from build123d import *

# Parameters (mm, degrees)
SKETCH1_W           = 100
SKETCH1_H           = 80
BOSS_EXTRUDE1_DEPTH = 5
SKETCH2_R           = 8.0125
CUT_EXTRUDE1_DEPTH  = 129.16005618
BOSS_EXTRUDE2_START = 45
SKETCH3_R           = 20.715
SKETCH3_R_2         = 8.0125
BOSS_EXTRUDE2_DEPTH = 45
SKETCH4_R           = 2.0193
CUT_EXTRUDE2_DEPTH  = 15
SKETCH6_R           = 2.0193
CUT_EXTRUDE3_DEPTH  = 15
SKETCH7_R           = 7.9375
CUT_EXTRUDE4_DEPTH  = 136.738719638


with BuildPart() as part:
    # Sketch1 → Boss-Extrude1 (new body)
    with BuildSketch(Plane(origin=(0, 0, 0), x_dir=(1, 0, 0), z_dir=(0, 1, 0))):
        with Locations((50, -40)):
            Rectangle(SKETCH1_W, SKETCH1_H)
    extrude(amount=BOSS_EXTRUDE1_DEPTH)

    # Sketch2 → Cut-Extrude1 (cut, through all)
    with BuildSketch(Plane(origin=(0, 5, 0), x_dir=(1, 0, 0), z_dir=(0, 1, 0))):
        with Locations(Location((50, -40, 0), (0, 0, 270))):
            Circle(SKETCH2_R)
    extrude(amount=-CUT_EXTRUDE1_DEPTH, mode=Mode.SUBTRACT)

    # Sketch3 → Boss-Extrude2 (add)
    with BuildSketch(Plane(origin=(0, 5, 0), x_dir=(1, 0, 0), z_dir=(0, 1, 0)).offset(BOSS_EXTRUDE2_START)):
        with Locations(Location((50, -40, 0), (0, 0, 90))):
            Circle(SKETCH3_R)
        with Locations(Location((50, -40, 0), (0, 0, 270))):
            Circle(SKETCH3_R_2, mode=Mode.SUBTRACT)
    extrude(amount=-BOSS_EXTRUDE2_DEPTH)

    # Sketch4 → Cut-Extrude2 (cut)
    with BuildSketch(Plane(origin=(63.180969698, 50, 55.980402461), x_dir=(0.7714411036002745, 0, -0.6363007336755088), z_dir=(0.6363007336755088, 0, 0.7714411036002745))):
        with Locations((0, -10)):
            Circle(SKETCH4_R)
        with Locations((0, -35)):
            Circle(SKETCH4_R)
    extrude(amount=-CUT_EXTRUDE2_DEPTH, mode=Mode.SUBTRACT)

    # Sketch6 → Cut-Extrude3 (cut)
    with BuildSketch(Plane(origin=(52.5543225, 0, -17.601285723), x_dir=(0, -1, 0), z_dir=(0.9482321037380778, 0, -0.3175781438330723))):
        with Locations(Location((-40, -53.808191341, 0), (0, 0, 90))):
            Circle(SKETCH6_R)
        with Locations(Location((-15, -53.808191341, 0), (0, 0, 90))):
            Circle(SKETCH6_R)
    extrude(amount=-CUT_EXTRUDE3_DEPTH, mode=Mode.SUBTRACT)

    # Sketch7 → Cut-Extrude4 (cut, through all)
    with BuildSketch(Plane(origin=(0, 5, 0), x_dir=(1, 0, 0), z_dir=(0, 1, 0))):
        with Locations(Location((84.125, -64.125, 0), (0, 0, 270))):
            Circle(SKETCH7_R)
        with Locations(Location((15.875, -64.125, 0), (0, 0, 270))):
            Circle(SKETCH7_R)
        with Locations(Location((15.875, -15.875, 0), (0, 0, 270))):
            Circle(SKETCH7_R)
        with Locations(Location((84.125, -15.875, 0), (0, 0, 270))):
            Circle(SKETCH7_R)
    extrude(amount=-CUT_EXTRUDE4_DEPTH, mode=Mode.SUBTRACT)


solid = part.part
Can you work these out from the model? Positions are in its coordinate system, mm. A direction names the side the tool comes from. Round coordinates to 2 decimals unless told otherwise and drop trailing zeros. Write each loop counter-clockwise with the first axis right and the second up, starting at its lowest first coordinate (ties: lowest second). Pieces come first, ordered by that corner, then holes. Notation, with made-up numbers: (25.5, 79.25) -> (33.5, 79.25) arc R11 cw to (33.5, 88.25) -> close; hole circle Ø4 at (51, 57). An arc over 180 degrees is marked (long way). One line per question, with ' | ' between items. Start each with the question number.
1) I need wall thicknesses on line 1 (X direction, y = 12.5, z = 40) (1 decimal); line 2 (Z direction, x = 84.5, y = 3); line 3 (Z direction, x = 12.5, y = 3). Which ranges of each line are inside material? Lowest first, please. Write a range as [from, to].
2) Suppose I cut it at A-A on x = 50. Write out the boundary of the cut face in (y, z) (1 decimal).
3) If we mould it in two halves opening along Z, with no side actions, what happens to faces 1 (the cylindrical face through (64.221, 15.089, 37.365)), 2 (the flat face through (49, 2, 0)), 3 (the flat face through (49, 0, 31))? For each: released by +Z, released by -Z, zero draft, split by the parting line, or undercut.
4) I'm going to push flat-ended pins straight in: P1, Ø20.5, axis at x = 84.125, z = 15.875, coming from the +Y side; P2, Ø1, axis at y = 26, z = 52, coming from the -X side; P3, Ø6, axis at y = 24, z = 33, coming from the -X side. Where does each tip first touch, or does it pass through?
5) Suppose I cut it at B-B on z = 10. Write out the boundary of the cut face in (x, y), then the cut area to 3 significant figures.
6) Suppose I cut it at D-D on x = 88. Write out the boundary of the cut face in (y, z).
7) Suppose I cut it at C-C on y = 35.5. Write out the boundary of the cut face in (x, z) (1 decimal).
8) On a 3-axis mill with a long thin cutter (end or side, diameter ignored), from which of +Z, -Z, +X, -X, +Y, -Y can I reach the whole of each face in a straight line? I mean faces 4 (the cylindrical face through (68.378, 27.815, 30.441)), 5 (the flat face through (49, 2, 80)). Say none if no direction works.
Return value:
1) line 1: x = [29.3, 42], [58, 70.7] | line 2: z = [0, 7.95], [23.8, 56.2], [72.05, 80] | line 3: z = [0, 8.69], [23.06, 56.94], [71.31, 80]
2) outline: (0, 0) -> (5, 0) -> (5, 19.3) -> (50, 19.3) -> (50, 32) -> (0, 32) -> close; (0, 48) -> (50, 48) -> (50, 60.7) -> (5, 60.7) -> (5, 80) -> (0, 80) -> close
3) face 1: undercut | face 2: released by -Z | face 3: zero draft
4) P1: stops at y = 5 | P2: stops at x = 32.77 | P3: stops at x = 29.67
5) outline: (0, 0) -> (10.54, 0) -> (10.54, 5) -> (0, 5) -> close; (21.21, 0) -> (78.79, 0) -> (78.79, 5) -> (21.21, 5) -> close; (89.46, 0) -> (100, 0) -> (100, 5) -> (89.46, 5) -> close | area: 393 mm2
6) outline: (0, 0) -> (5, 0) -> (5, 8.95) -> (0, 8.95) -> close; (0, 22.8) -> (5, 22.8) -> (5, 57.2) -> (0, 57.2) -> close; (0, 71.05) -> (5, 71.05) -> (5, 80) -> (0, 80) -> close
7) outline: circle Ø41.4 at (50, 40); hole circle Ø16 at (50, 40)
8) face 4: +Y | face 5: +Z, +X, -X, +Y, -Y
